from build123d import *

# Parameters (mm, degrees)
BOSS_EXTRUDE1_DEPTH = 15
SKETCH3_R           = 1.5
CUT_EXTRUDE1_DEPTH  = 15


with BuildPart() as part:
    # Sketch2 → Boss-Extrude1 (new body)
    with BuildSketch(Plane(origin=(0, 0, 0), x_dir=(0, 0, -1), z_dir=(1, 0, 0))):
        with BuildLine():
            Line((-22.89893617, 5), (7.10106383, 5))
            Line((7.10106383, 5), (52.738984118, -49.389155461))
            ThreePointArc((52.738984118, -49.389155461), (63.539400353, -65.918178681), (48.089840145, -53.623111018))
            Line((48.089840145, -53.623111018), (3.094707467, 0))
            Line((3.094707467, 0), (-22.89893617, 0))
            Line((-22.89893617, 0), (-22.89893617, 5))
        make_face()
    extrude(amount=-BOSS_EXTRUDE1_DEPTH)

    # Sketch3 → Cut-Extrude1 (cut)
    with BuildSketch(Plane(origin=(0, 5, 0), x_dir=(1, 0, 0), z_dir=(0, 1, 0))):
        with Locations((-7.417246122, 0)):
            Circle(SKETCH3_R)
        with Locations((-7.417246122, -15.103846838)):
            Circle(SKETCH3_R)
    extrude(amount=-CUT_EXTRUDE1_DEPTH, mode=Mode.SUBTRACT)


solid = part.part
The model under review builds one solid part; all positions refer to its coordinate system, in mm. A direction names the side the tool comes from. Round coordinates to 2 decimals unless told otherwise and drop trailing zeros. Write each loop counter-clockwise with the first axis right and the second up, starting at its lowest first coordinate (ties: lowest second). Pieces come first, ordered by that corner, then holes. Notation, with made-up numbers: M 38.25,31.25 L 91.25,31.25 A17 cw 91.25,36.25 Z; hole C 73,-19.75 d5. An arc over 180 degrees is marked long. Use a Markdown table: item, result. Add a question column.
Q1. We need section C-C, the plane z = 9.5. State the section outline as (x, y) points.
Q2. We need section A-A, the plane z = 0. State the section outline as (x, y) points.
Q3. Machinability: for faces 5 (the face through (-7, 0, 10)), 6 (the face through (-7, 5, 8)), which of the approach directions +Z, -Z, +X, -X, +Y, -Y give a long, thin tool a straight path to every point of the face, cutting with its end or side? Answer none if there is none.
Q4. We need section D-D, the plane y = -38. State the section outline as (x, z) points.
Q5. The part is to be moulded in two halves that separate along X. For faces 1 (the face through (-8.523, 2.535, 14.09)), 2 (the face through (0, -32, -32)), 3 (the face through (-8.916, 2.535, -0.066)), 4 (the face through (-7.395, -21.814, -29.601)), say which applies: pulls with the +X half, pulls with the -X half, needs draft (parallel to the pull), parting line crosses it, or undercut.
Q6. Insertion check: pin 1 (2 mm diameter, centred on x = -5.5, y = -17, fed in from -Z); pin 2 (6 mm diameter, centred on x = -10.5, z = -28, fed in from -Y); pin 3 (1 mm diameter, centred on x = -12.5, z = -11.5, fed in from -Y); pin 4 (3 mm diameter, centred on y = -47, z = -55, fed in from +X). Each pin has a flat end and moves straight along its axis. Give the tip position at first contact, or say it passes through.
Q7. We need section B-B, the plane x = -3.5. State the section outline as (y, z) points.
Q8. To check wall thickness, follow line 1 (Y direction, x = -7.5, z = 7.5); line 2 (Y direction, x = -11, z = -33); line 3 (Z direction, x = -9.5, y = -33) (3 decimals). State the ranges of each line that lie inside material, in increasing order.
Findings below:
| question | item | result |
|---|---|---|
| 1 | outline | M -15,0 L 0,0 L 0,5 L -15,5 Z |
| 2 | outline | M -15,0 L -8.92,0 L -8.92,5 L -15,5 Z; M -5.92,0 L 0,0 L 0,5 L -5.92,5 Z |
| 3 | face 5 | +Z, +X, -X, -Y |
| 3 | face 6 | +Z, -Z, +X, -X, +Y |
| 4 | outline | M -15,-43.18 L 0,-43.18 L 0,-34.98 L -15,-34.98 Z |
| 5 | face 1 | undercut |
| 5 | face 2 | pulls with the +X half |
| 5 | face 3 | undercut |
| 5 | face 4 | needs draft |
| 6 | pin 1 | stops at z = -26.4 |
| 6 | pin 2 | stops at y = -33.26 |
| 6 | pin 3 | stops at y = -10.61 |
| 6 | pin 4 | passes through |
| 7 | outline | M -53.62,-48.09 A10 ccw long -49.39,-52.74 L 5,-7.1 L 5,22.9 L 0,22.9 L 0,-3.09 Z |
| 8 | line 1 | y = 0 to 5 |
| 8 | line 2 | y = -35.64 to -25.87 |
| 8 | line 3 | z = -38.987 to -30.785 |
